from build123d import *

# Parameters (mm, degrees)
SKETCH2_R               = 4.953
SKETCH2_W               = 64
SKETCH2_H               = 48.5
BOSS_EXTRUDE1_DEPTH     = 72.4
BOSS_EXTRUDE3_DEPTH     = 1
SKETCH3_4_R             = 7.493
BOSS_EXTRUDE4_DEPTH     = 12.4
SKETCH6_R               = 6.993
CUT_EXTRUDE1_DEPTH      = 12.4
BOSS_EXTRUDE5_DEPTH     = 25
BOSS_EXTRUDE6_START     = 25
SKETCH7_R               = 4.953
BOSS_EXTRUDE6_DEPTH     = 25
CUT_EXTRUDE2_DEPTH      = 120.245838502
CUT_EXTRUDE2_DEPTH_BACK = 120.245838502
SKETCH8_W               = 16
SKETCH8_H               = 1.27


with BuildPart() as part:
    # Sketch2 → Boss-Extrude1 (new body)
    with BuildSketch(Plane(origin=(0, 0, 0), x_dir=(0, 0, -1), z_dir=(1, 0, 0))):
        with Locations((0, -24.25)):
            Circle(SKETCH2_R)
        Rectangle(SKETCH2_W, SKETCH2_H)
        with BuildLine():
            Line((32, -24.25), (-32, -24.25))
            ThreePointArc((-32, -24.25), (0, -56.25), (32, -24.25))
        make_face()
        with BuildLine():
            ThreePointArc((-4.953, -24.25), (0, -29.203), (4.953, -24.25))
            Line((4.953, -24.25), (-4.953, -24.25))
        make_face()
        with BuildLine():
            Line((-4.953, -24.25), (4.953, -24.25))
            ThreePointArc((4.953, -24.25), (0, -19.297), (-4.953, -24.25))
        make_face()
    extrude(amount=-BOSS_EXTRUDE1_DEPTH)

    # Sketch3 → Boss-Extrude3 (add)
    with BuildSketch(Plane(origin=(0, 24.25, 0), x_dir=(1, 0, 0), z_dir=(0, 1, 0))):
        Polygon((-57.9126, -9.1313), (-55.1313, -11.9126), (-36.8687, -11.9126), (-34.0874, -9.1313), (-34.0874, 9.1313), (-36.8687, 11.9126), (-55.1313, 11.9126), (-57.9126, 9.1313), align=None)
    extrude(amount=BOSS_EXTRUDE3_DEPTH)

    # Sketch3_4 → Boss-Extrude4 (add)
    with BuildSketch(Plane(origin=(0, 24.25, 0), x_dir=(1, 0, 0), z_dir=(0, 1, 0))):
        with Locations(Location((-46, 0, 0), (0, 0, 90))):
            Circle(SKETCH3_4_R)
    extrude(amount=BOSS_EXTRUDE4_DEPTH)

    # Sketch6 → Cut-Extrude1 (cut)
    with BuildSketch(Plane(origin=(0, 36.65, 0), x_dir=(1, 0, 0), z_dir=(0, 1, 0))):
        with Locations(Location((-46, 0, 0), (0, 0, 270))):
            Circle(SKETCH6_R)
    extrude(amount=-CUT_EXTRUDE1_DEPTH, mode=Mode.SUBTRACT)

    # Sketch2_3 → Boss-Extrude5 (add)
    with BuildSketch(Plane(origin=(0, 0, 0), x_dir=(0, 0, -1), z_dir=(1, 0, 0))):
        with BuildLine():
            ThreePointArc((-4.953, -24.25), (0, -29.203), (4.953, -24.25))
            Line((4.953, -24.25), (-4.953, -24.25))
        make_face()
        with BuildLine():
            Line((-4.953, -24.25), (4.953, -24.25))
            ThreePointArc((4.953, -24.25), (0, -19.297), (-4.953, -24.25))
        make_face()
    extrude(amount=BOSS_EXTRUDE5_DEPTH)

    # Sketch7 → Boss-Extrude6 (add)
    with BuildSketch(Plane.ZY.offset(72.4).offset(BOSS_EXTRUDE6_START)):
        with Locations(Location((0, -24.25, 0), (0, 0, 180))):
            Circle(SKETCH7_R)
    extrude(amount=-BOSS_EXTRUDE6_DEPTH)

    # Sketch8 → Cut-Extrude2 (cut, two sides: drawn at the far end of the back side and taken through both)
    with BuildSketch(Plane(origin=(0, -24.25, 0), x_dir=(1, 0, 0), z_dir=(0, 1, 0)).offset(-CUT_EXTRUDE2_DEPTH_BACK)):
        with Locations((17, -4.318)):
            Rectangle(SKETCH8_W, SKETCH8_H)
        with Locations((-89.4, -4.318)):
            Rectangle(SKETCH8_W, SKETCH8_H)
    extrude(amount=CUT_EXTRUDE2_DEPTH + CUT_EXTRUDE2_DEPTH_BACK, mode=Mode.SUBTRACT)


solid = part.part
Verification items for the finished model (mm, model axes). A direction names the side the tool comes from. Give positions to 0.01 mm unless a question says otherwise; leave off trailing zeros. Loops run counter-clockwise (first coordinate to the right, second up) from the corner with the lowest first, then second, coordinate; pieces in that order, holes last.
1) Thickness scan on line 1 along X through (y, z) = (32.25, 0); line 2 along X through (y, z) = (-6, 0.5); line 3 along Y through (x, z) = (-28.5, -1). Record the ranges inside material, lowest first.
2) Sectioned sample at C-C, the plane y = 14.5. Enter the section's corners in (x, z).
3) Sectioned sample at A-A, the plane x = -46. Enter the section's corners in (y, z).
4) Sectioned sample at B-B, the plane z = 0. Enter the section's corners in (x, y), then the cut area to 3 significant figures.
5) Sectioned sample at D-D, the plane x = -2. Enter the section's corners in (y, z).
6) Set-up check for faces 4 (the cylindrical face through (-85.075, -25.738, -4.724)), 5 (the flat face through (-35.498, 24.743, 10.541)), 6 (the flat face through (-35.459, 24.743, -10.502)), 7 (the cylindrical face through (-39.352, 30.87, -3.458)): record each of +Z, -Z, +X, -X, +Y, -Y from which the full face is reachable in a straight line by a thin tool's end or side.
7) Depth check by flat-ended pin: pin 1 Ø5.5 at (x, y) = (19.5, -24.5) entering from +Z; pin 2 Ø6 at (y, z) = (-5, 18) entering from +X; pin 3 Ø2 at (y, z) = (-33, 4.5) entering from -X; pin 4 Ø4 at (x, z) = (11, -7) entering from +Y. Enter the tip coordinate at first touch or a pass-through.
8) Draft check along X on faces 1 (the cylindrical face through (-52.827, 30.537, -1.516)), 2 (the flat face through (-72.4, -15, 0)), 3 (the flat face through (-36, 0, -32)). Enter one of: pulls with the +X half, pulls with the -X half, needs draft (parallel to the pull), parting line crosses it, or undercut.
Answers:
1. line 1: x = -53.49 to -52.99, -39.01 to -38.51
1. line 2: x = -72.4 to 0
1. line 3: y = -56.23 to 24.25
2. outline: (-72.4, -32) - (0, -32) - (0, 32) - (-72.4, 32) - close
3. outline: (-24.25, -32) - (24.25, -32) - (24.25, -11.91) - (25.25, -11.91) - (25.25, -7.49) - (36.65, -7.49) - (36.65, -6.99) - (24.25, -6.99) - (24.25, 6.99) - (36.65, 6.99) - (36.65, 7.49) - (25.25, 7.49) - (25.25, 11.91) - (24.25, 11.91) - (24.25, 32) - (-24.25, 32) arc R32 ccw to start
4. outline: (-97.4, -29.2) - (-72.4, -29.2) - (-72.4, -56.25) - (0, -56.25) - (0, -29.2) - (25, -29.2) - (25, -19.3) - (0, -19.3) - (0, 24.25) - (-34.09, 24.25) - (-34.09, 25.25) - (-38.51, 25.25) - (-38.51, 36.65) - (-39.01, 36.65) - (-39.01, 24.25) - (-52.99, 24.25) - (-52.99, 36.65) - (-53.49, 36.65) - (-53.49, 25.25) - (-57.91, 25.25) - (-57.91, 24.25) - (-72.4, 24.25) - (-72.4, -19.3) - (-97.4, -19.3) - close
4. area: 6,340 mm2
5. outline: (-24.25, -32) - (24.25, -32) - (24.25, 32) - (-24.25, 32) arc R32 ccw to start
6. face 4: -X
6. face 5: +Z, +X, +Y
6. face 6: -Z, +X, +Y
6. face 7: +Y
7. pin 1: stops at z = 3.68
7. pin 2: stops at x = 0
7. pin 3: stops at x = -72.4
7. pin 4: passes through
8. face 1: undercut
8. face 2: pulls with the -X half
8. face 3: needs draft
